Build history of the part. All positions in model axes, mm. Face numbers are marked on the shaded views. A direction names the side the tool comes from. Give positions to 0.01 mm unless a question says otherwise; leave off trailing zeros. Loops run counter-clockwise (first coordinate to the right, second up) from the corner with the lowest first, then second, coordinate; pieces in that order, holes last. Notation, with made-up numbers: M 33.25,79.25 L 58.25,79.25 A27 ccw 58.25,107.25 Z; hole C 47.5,73 d1. An arc over 180 degrees is marked long. Put each result on its own line as item: value.
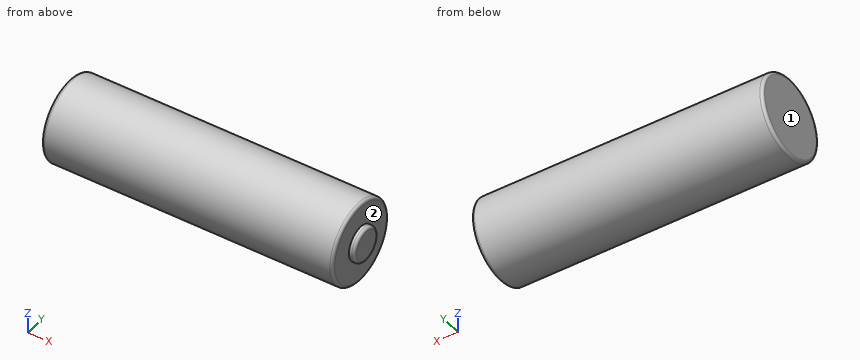
```python
from build123d import *

# Parameters (mm, degrees)
SKETCH1_R           = 7.17
BOSS_EXTRUDE1_DEPTH = 25.5
SKETCH2_R           = 3
BOSS_EXTRUDE2_DEPTH = 1
FILLET1_R           = 0.5


with BuildPart() as part:
    # Sketch1 → Boss-Extrude1 (new, symmetric)
    with BuildSketch(Plane(origin=(0, 0, 0), x_dir=(0, 0, -1), z_dir=(1, 0, 0))):
        Circle(SKETCH1_R)
    extrude(amount=BOSS_EXTRUDE1_DEPTH, both=True)

    # Sketch2 → Boss-Extrude2 (add)
    with BuildSketch(Plane(origin=(25.5, 0, 0), x_dir=(0, 0, -1), z_dir=(1, 0, 0))):
        Circle(SKETCH2_R)
    extrude(amount=BOSS_EXTRUDE2_DEPTH)

    # Fillet1
    fillet1_edges = [part.edges().sort_by_distance(p)[0] for p in [
        (-25.5, 0, 7.17),
        (25.5, 0, 7.17),
        (26.5, 0, 3),
    ]]
    fillet(fillet1_edges, radius=FILLET1_R)


solid = part.part
```
Q1. Tool access for the marked faces 1 and 2: list every direction of +Z, -Z, +X, -X, +Y, -Y with a clear straight run to the whole face (end or side of a thin tool).
Here are the results:
face 1: +Z, -Z, -X, +Y, -Y
face 2: +X
Q2. Probe line 1 (X direction, y = -0.25, z = -3.5); line 2 (Z direction, x = 16, y = 0.25); line 3 (Y direction, x = 15, z = 0.5). List the from-to ranges inside material, lowest first. Write a range as from..to.
Here are the results:
line 1: -25.5..25.5
line 2: -7.17..7.17
line 3: -7.15..7.15
Q3. Drop flat-ended pins along their axis: pin 1 Ø2 at (x, y) = (17, 5) entering from +Z; pin 2 Ø6 at (x, y) = (-8.5, -4) entering from +Z; pin 3 Ø2 at (x, y) = (2, 1.5) entering from +Z. Give the stop position or say it passes through.
Here are the results:
pin 1: z = 5.95
pin 2: z = 7.1
pin 3: z = 7.15
Q4. Slice it at A-A (x = 9.5). List the corners of the cut face in (y, z).
Here are the results:
outline: C 0,0 d14.34
